Build history of the part. All positions in model axes, mm. A direction names the side the tool comes from. Round coordinates to 2 decimals unless told otherwise and drop trailing zeros. Write each loop counter-clockwise with the first axis right and the second up, starting at its lowest first coordinate (ties: lowest second). Pieces come first, ordered by that corner, then holes. Notation, with made-up numbers: M 44.25,16 L 98.25,16 A18 ccw 98.25,35 Z; hole C 43.5,51 d1. An arc over 180 degrees is marked long. Write item = value, one per line. Start each with the question number.
Q1. Band-saw the part on A-A on z = 1.4. Write the cut outline in (x, y).
Q2. Probe L1, parallel to Y at x = -0.25, z = 1.7; L2, parallel to Y at x = -9, z = 0.8; L3, parallel to X at y = 32, z = 2.85. List the from-to ranges inside material, lowest first.
Q3. Drop a flat-ended pin along its axis: P1, Ø1.5, axis at y = 25, z = 2, coming from the -X side. Give the stop position or say it passes through.
Q4. Band-saw the part on B-B on x = 5.25. Write the cut outline in (y, z), plus the area to 3 significant figures.
Q5. Tool access for faces 4 (the flat face through (-9, 34.051, 1)), 5 (the flat face through (9.796, 19, 1)): list every direction of +Z, -Z, +X, -X, +Y, -Y with a clear straight run to the whole face (end or side of a thin tool).
Q6. Band-saw the part on C-C on y = 13. Write the cut outline in (x, z).
Q7. Pull direction X, two halves, no side cores. Call faces 1 (the cylindrical face through (-0.37, 45.29, 1.52)), 2 (the cylindrical face through (6.944, 51.044, 1.521)), 3 (the flat face through (-5, 54.051, 1)): released by +X, released by -X, zero draft, split by the parting line, or undercut.
```python
from build123d import *

# Parameters (mm, degrees)
SKETCH_1_W          = 20
SKETCH_1_H          = 69
EXTRUDE_1_DEPTH     = 3
SKETCH_2_W          = 3
SKETCH_2_H          = 29
CUT_EXTRUDE_1_DEPTH = 3
HOLE_WIZARD_M3_1_D  = 2.5
FILLET_1_R          = 10


with BuildPart() as part:
    # 草图1 → 凸台-拉伸1 (new body)
    with BuildSketch(Plane.XY):
        with Locations((-0.204081633, 19.551020408)):
            Rectangle(SKETCH_1_W, SKETCH_1_H)
    extrude(amount=EXTRUDE_1_DEPTH)

    # 草图2 → 切除-拉伸1 (cut)
    with BuildSketch(Plane.XY):
        with Locations((-8.704081633, 19.551020408)):
            Rectangle(SKETCH_2_W, SKETCH_2_H)
    extrude(amount=CUT_EXTRUDE_1_DEPTH, mode=Mode.SUBTRACT)

    # M3 螺纹孔的螺纹孔钻头1 (through all)
    with Locations(Plane(origin=(0, 0, 0), x_dir=(-1, 0, 0), z_dir=(0, 0, -1))):
        with Locations((0.204081633, 44.051020408), (0.204081633, -4.948979592)):
            Hole(HOLE_WIZARD_M3_1_D / 2)

    # 圆角1
    fillet_1_edges = [part.edges().sort_by_distance(p)[0] for p in [
        (9.795918367, 54.051020408, 1.5),
        (9.795918367, -14.948979592, 1.5),
    ]]
    fillet(fillet_1_edges, radius=FILLET_1_R)


solid = part.part
```
Conclusion:
q1.outline = M -10.2,-14.95 L -0.2,-14.95 A10 ccw 9.8,-4.95 L 9.8,44.05 A10 ccw -0.2,54.05 L -10.2,54.05 L -10.2,34.05 L -7.2,34.05 L -7.2,5.05 L -10.2,5.05 Z; hole C -0.2,-4.95 d2.5; hole C -0.2,44.05 d2.5
q2.L1 = -14.95 to -6.2, -3.7 to 42.8, 45.3 to 54.05
q2.L2 = -14.95 to 5.05, 34.05 to 54.05
q2.L3 = -7.2 to 9.8
q3.P1 = -7.2
q4.outline = M -13.33,0 L 52.43,0 L 52.43,3 L -13.33,3 Z
q4.area = 197 mm^2
q5.face_4 = +Z, -Z, -X
q5.face_5 = +Z, -Z, +X, +Y, -Y
q6.outline = M -7.2,0 L 9.8,0 L 9.8,3 L -7.2,3 Z
q7.face_1 = undercut
q7.face_2 = released by +X
q7.face_3 = zero draft
